```python
from build123d import *

# Parameters (mm, degrees)
SKETCH4_W                      = 69.85
SKETCH4_H                      = 127
BOSS_EXTRUDE4_DEPTH            = 6.35
CBORE_FOR_M3_SHCS1_D           = 3.4
CBORE_FOR_M3_SHCS1_CBORE_D     = 6.5
CBORE_FOR_M3_SHCS1_CBORE_DEPTH = 3.5
SKETCH7_R                      = 1.651
CUT_EXTRUDE1_DEPTH             = 73.748389157
SKETCH16_W                     = 12.7
SKETCH16_H                     = 63.5
BOSS_EXTRUDE6_DEPTH            = 50.8
SKETCH18_W                     = 6.35
SKETCH18_H                     = 63.5
BOSS_EXTRUDE7_DEPTH            = 44.45
CUT_EXTRUDE3_REACH             = 94.294
SKETCH21_R                     = 11.25
CBORE_START                    = 54.15
CBORE_FOR_M3_SHCS3_OUTLINE_R   = 3.25
CBORE_FOR_M3_SHCS3_DEPTH       = 3
CBORE_START_2                  = 50.8
CBORE_FOR_M3_SHCS3_2_OUTLINE_R = 1.7
CBORE_FOR_M3_SHCS3_2_DEPTH     = 3.35
CBORE_FOR_M3_SHCS3_3_OUTLINE_R = 1.7
CBORE_FOR_M3_SHCS3_3_DEPTH     = 6.35
CUT_EXTRUDE5_REACH             = 94.294
CUT_EXTRUDE6_REACH             = 90.502
SKETCH24_W                     = 42.188209008
SKETCH24_H                     = 6.56852392
SKETCH25_W                     = 19.05
SKETCH25_H                     = 40.64
BOSS_EXTRUDE8_DEPTH            = 35.548437
BOSS_EXTRUDE9_DEPTH            = 5
SKETCH32_W                     = 8.128
SKETCH32_H                     = 38.354
CUT_EXTRUDE8_DEPTH             = 1.524
M3_CLEARANCE_HOLE2_D           = 2.8
FILLET6_R                      = 2.54
FILLET9_R                      = 2
FILLET10_R                     = 2
FILLET11_R                     = 2


# Read off the part's stored shape, not the designer's step: CBORE for M3 SHCS3
with BuildPart() as part:
    # Sketch4 → Boss-Extrude4 (new body)
    with BuildSketch(Plane.XY):
        Rectangle(SKETCH4_W, SKETCH4_H)
    extrude(amount=BOSS_EXTRUDE4_DEPTH)

    # CBORE for M3 SHCS1 (through all)
    with Locations(Plane.XY.offset(6.35)):
        with Locations((-10, -24.45), (10, -44.45), (10, -24.45), (-10, -44.45)):
            CounterBoreHole(CBORE_FOR_M3_SHCS1_D / 2, CBORE_FOR_M3_SHCS1_CBORE_D / 2, CBORE_FOR_M3_SHCS1_CBORE_DEPTH)

    # Sketch7 → Cut-Extrude1 (cut, through all)
    with BuildSketch(Plane.XY.offset(6.35)):
        with Locations((-12.5, -34.45)):
            Circle(SKETCH7_R)
        with Locations((12.5, -34.45)):
            Circle(SKETCH7_R)
    extrude(amount=-CUT_EXTRUDE1_DEPTH, mode=Mode.SUBTRACT)

    # Sketch16 → Boss-Extrude6 (add)
    with BuildSketch(Plane.XY.offset(6.35)):
        with Locations((-28.575, 31.75)):
            Rectangle(SKETCH16_W, SKETCH16_H)
        with Locations((28.575, 31.75)):
            Rectangle(SKETCH16_W, SKETCH16_H)
    extrude(amount=BOSS_EXTRUDE6_DEPTH)

    # Sketch18 → Boss-Extrude7 (add)
    with BuildSketch(Plane(origin=(-22.225, 0, 0), x_dir=(0, 0, -1), z_dir=(1, 0, 0))):
        with Locations((-53.975, 31.75)):
            Rectangle(SKETCH18_W, SKETCH18_H)
    extrude(amount=BOSS_EXTRUDE7_DEPTH)

    # Sketch21 → Cut-Extrude3 (cut, up to next)
    with BuildSketch(Plane.XY.offset(57.15), mode=Mode.PRIVATE) as cut_extrude3_sk1:
        with Locations((0, 31.75)):
            Circle(SKETCH21_R)
    cut_extrude3_tool1 = extrude(cut_extrude3_sk1.sketch, amount=-CUT_EXTRUDE3_REACH, mode=Mode.PRIVATE) & part.part
    add(cut_extrude3_tool1.solids().sort_by_distance((0, 31.75, 57.15))[0], mode=Mode.SUBTRACT)

    # CBORE for M3 SHCS3 outline → CBORE for M3 SHCS3 (cut)
    with BuildSketch(Plane.XY.offset(CBORE_START)):
        with Locations((-15.5, 47.25)):
            Circle(CBORE_FOR_M3_SHCS3_OUTLINE_R)
        with Locations((-15.5, 16.25)):
            Circle(CBORE_FOR_M3_SHCS3_OUTLINE_R)
        with Locations((15.5, 47.25)):
            Circle(CBORE_FOR_M3_SHCS3_OUTLINE_R)
        with Locations((15.5, 16.25)):
            Circle(CBORE_FOR_M3_SHCS3_OUTLINE_R)
    extrude(amount=CBORE_FOR_M3_SHCS3_DEPTH, mode=Mode.SUBTRACT)

    # CBORE for M3 SHCS3 2 outline → CBORE for M3 SHCS3 2 (cut)
    with BuildSketch(Plane.XY.offset(CBORE_START_2)):
        with Locations((-15.5, 47.25)):
            Circle(CBORE_FOR_M3_SHCS3_2_OUTLINE_R)
        with Locations((-15.5, 16.25)):
            Circle(CBORE_FOR_M3_SHCS3_2_OUTLINE_R)
        with Locations((15.5, 47.25)):
            Circle(CBORE_FOR_M3_SHCS3_2_OUTLINE_R)
        with Locations((15.5, 16.25)):
            Circle(CBORE_FOR_M3_SHCS3_2_OUTLINE_R)
    extrude(amount=CBORE_FOR_M3_SHCS3_2_DEPTH, mode=Mode.SUBTRACT)

    # CBORE for M3 SHCS3 3 outline → CBORE for M3 SHCS3 3 (cut)
    with BuildSketch(Plane.XY):
        with Locations((0, 31.75)):
            Circle(CBORE_FOR_M3_SHCS3_3_OUTLINE_R)
    extrude(amount=CBORE_FOR_M3_SHCS3_3_DEPTH, mode=Mode.SUBTRACT)

    # Sketch23 → Cut-Extrude5 (cut, up to next)
    with BuildSketch(Plane.XY.offset(57.15), mode=Mode.PRIVATE) as cut_extrude5_sk1:
        with BuildLine():
            Line((-2.53747066, 36.810770012), (-2.53747066, 63.5))
            ThreePointArc((-2.53747066, 63.5), (0, 66.03747066), (2.53747066, 63.5))
            Line((2.53747066, 63.5), (2.53747066, 36.810770012))
            ThreePointArc((2.53747066, 36.810770012), (0, 34.273299352), (-2.53747066, 36.810770012))
        make_face()
    cut_extrude5_tool1 = extrude(cut_extrude5_sk1.sketch, amount=-CUT_EXTRUDE5_REACH, mode=Mode.PRIVATE) & part.part
    add(cut_extrude5_tool1.solids().sort_by_distance((0, 50.155385, 57.15))[0], mode=Mode.SUBTRACT)

    # Sketch24 → Cut-Extrude6 (cut, up to next)
    with BuildSketch(Plane.XY.offset(6.35), mode=Mode.PRIVATE) as cut_extrude6_sk1:
        Rectangle(SKETCH24_W, SKETCH24_H)
    cut_extrude6_tool1 = extrude(cut_extrude6_sk1.sketch, amount=-CUT_EXTRUDE6_REACH, mode=Mode.PRIVATE) & part.part
    add(cut_extrude6_tool1.solids().sort_by_distance((0, 0, 6.35))[0], mode=Mode.SUBTRACT)

    # Sketch25 → Boss-Extrude8 (add)
    with BuildSketch(Plane.ZY.offset(34.925)):
        with Locations((12.777, 31.75)):
            Rectangle(SKETCH25_W, SKETCH25_H)
    extrude(amount=BOSS_EXTRUDE8_DEPTH)

    # Sketch31 → Boss-Extrude9 (add, symmetric)
    with BuildSketch(Plane(origin=(0, 0, 12.777), x_dir=(-1, 0, 0), z_dir=(0, 0, -1))):
        Polygon((34.925, 11.43), (70.4734375, 11.43), (34.925, 0), align=None)
    extrude(amount=BOSS_EXTRUDE9_DEPTH, both=True)

    # Sketch32 → Cut-Extrude8 (cut)
    with BuildSketch(Plane.XY.offset(22.302)):
        with Locations((-55.4734375, 31.75)):
            Rectangle(SKETCH32_W, SKETCH32_H)
    extrude(amount=-CUT_EXTRUDE8_DEPTH, mode=Mode.SUBTRACT)

    # M3 Clearance Hole2 (through all)
    with Locations(Plane.XY.offset(20.778)):
        with Locations((-55.4734375, 31.75)):
            Hole(M3_CLEARANCE_HOLE2_D / 2)

    # Fillet6
    fillet6_edges = [part.edges().sort_by_distance(p)[0] for p in [
        (-34.925, 11.43, 5.5145),
        (-34.925, 11.43, 20.0395),
        (-52.699218512, 11.43, 17.777),
        (-52.699218512, 11.43, 7.777),
    ]]
    fillet(fillet6_edges, radius=FILLET6_R)

    # Fillet9
    # the kernel refuses this fillet: 2 mm, written as the material it takes off along each edge
    with BuildSketch(Plane(origin=(-70.473437, 57.07, 22.302), x_dir=(0, 0, -1), z_dir=(0, -1, 0)), Plane(origin=(-70.473437, 6.43, 3.252), x_dir=(0, 0, 1), z_dir=(0, 1, 0))) as fillet9_piece_1:
        with BuildLine():
            CenterArc((FILLET9_R, FILLET9_R), FILLET9_R, 180, 90)
            Line((0, FILLET9_R), (0, 0))
            Line((0, 0), (FILLET9_R, 0))
        make_face()
    extrude(amount=50.64, mode=Mode.SUBTRACT)
    with BuildSketch(Plane(origin=(-70.473437, 52.07, -1.748), x_dir=(0, -1, 0), z_dir=(0, 0, 1))) as fillet9_piece_2:
        with BuildLine():
            CenterArc((FILLET9_R, FILLET9_R), FILLET9_R, 180, 90)
            Line((0, FILLET9_R), (0, 0))
            Line((0, 0), (FILLET9_R, 0))
        make_face()
    extrude(amount=29.05, mode=Mode.SUBTRACT)

    # Fillet10
    fillet10_edges = [part.edges().sort_by_distance(p)[0] for p in [
        (-34.925, 52.07, 12.777),
    ]]
    fillet(fillet10_edges, radius=FILLET10_R)

    # Fillet11
    fillet11_edges = [part.edges().sort_by_distance(p)[0] for p in [
        (-34.925, 31.48, 3.252),
        (-34.925, 31.48, 22.302),
    ]]
    fillet(fillet11_edges, radius=FILLET11_R)


solid = part.part
```
CAD build for the part. Positions are in the model's coordinates, mm. A direction names the side the tool comes from. Coordinates: 2 decimals unless noted, no trailing zeros. Order: outer loops, then holes, each group sorted by start corner. A loop starts at its lowest first (then second) coordinate and runs counter-clockwise, first axis right, second up. Notation, with made-up numbers: (85, -3.75) - (103, -3.75) arc R25 cw to (103, 22.25) - close; hole circle Ø6 at (75.25, 80). An arc over 180 degrees is marked (long way). Answer in a Markdown table with one row per item.
1. Pull direction Y, two halves, no side cores. Call faces 1 (the face through (-13.247, -44.307, 4.624)), 2 (the face through (-22.225, 31, 28)), 3 (the face through (0, 0, 55)), 4 (the face through (8.43, -45.1, 1.41)): +Y half, -Y half, draft (parallel to the pull), parting line (faces both ways), or undercut.
Answer:
| item | result |
|---|---|
| face 1 | undercut |
| face 2 | draft |
| face 3 | -Y half |
| face 4 | undercut |
2. Flat gauge pins, fed straight in: P1, Ø2, axis at x = 0, z = 51.5, coming from the -Y side; P2, Ø4.5, axis at x = -48.5, y = 4.5, coming from the -Z side; P3, Ø5, axis at y = 51, z = 53.5, coming from the -X side (3 decimals). Where does each tip first touch, or does it go through?
Answer:
| item | result |
|---|---|
| P1 | y = 0 |
| P2 | z = 7.78 |
| P3 | x = -34.925 |
3. Slice it at C-C, the plane z = 35.5. List the corners of the cut face in (x, y) (3 decimals), then the cut area to 3 significant figures.
Answer:
| item | result |
|---|---|
| outline | (-34.925, 0) - (-22.225, 0) - (-22.225, 63.5) - (-34.925, 63.5) - close; (22.225, 0) - (34.925, 0) - (34.925, 63.5) - (22.225, 63.5) - close |
| area | 1,610 mm² |
4. Slice it at B-B, the plane x = 0. List the corners of the cut face in (y, z).
Answer:
| item | result |
|---|---|
| outline | (-63.5, 0) - (-3.28, 0) - (-3.28, 6.35) - (-63.5, 6.35) - close; (0, 50.8) - (20.5, 50.8) - (20.5, 57.15) - (0, 57.15) - close; (3.28, 0) - (30.05, 0) - (30.05, 6.35) - (3.28, 6.35) - close; (33.45, 0) - (63.5, 0) - (63.5, 6.35) - (33.45, 6.35) - close |
5. Drill centre lines: L1, parallel to Y at x = -15.5, z = 56.25; L2, parallel to Y at x = -10, z = 1; L3, parallel to X at y = 16, z = 55 (3 decimals). Where is each one in solid material? Low to high. Write a range as from..to.
Answer:
| item | result |
|---|---|
| L1 | 0..13, 19.5..44, 50.5..63.5 |
| L2 | -63.5..-46.15, -42.75..-26.15, -22.75..-3.28, 3.28..63.5 |
| L3 | -34.925..-18.74, -12.26..12.26, 18.74..34.925 |
6. Slice it at D-D, the plane y = 31.75. Give the number of separate pieces and of enclosed holes in the cut face, then the cut area to 3 significant figures.
Answer:
| item | result |
|---|---|
| separate pieces | 3 |
| enclosed holes | 0 |
| area | 2,470 mm² |
7. Slice it at A-A, the plane y = -24.45. List the corners of the cut face in (x, z) (3 decimals), then the cut area to 3 significant figures.
Answer:
| item | result |
|---|---|
| outline | (-34.925, 0) - (-11.7, 0) - (-11.7, 2.85) - (-13.25, 2.85) - (-13.25, 6.35) - (-34.925, 6.35) - close; (-8.3, 0) - (8.3, 0) - (8.3, 2.85) - (6.75, 2.85) - (6.75, 6.35) - (-6.75, 6.35) - (-6.75, 2.85) - (-8.3, 2.85) - close; (11.7, 0) - (34.925, 0) - (34.925, 6.35) - (13.25, 6.35) - (13.25, 2.85) - (11.7, 2.85) - close |
| area | 379 mm² |
8. 3-axis set-ups, long thin cutter, end or side, ignore diameter. For faces 5 (the face through (-21.094, 0, 3)), 6 (the face through (-43, 6, 7.777)), 7 (the face through (-52, 31, 3.252)), 8 (the face through (2.537, 53, 54)), 9 (the face through (17, 15, 54.15)): which of +Z, -Z, +X, -X, +Y, -Y reach the whole face in a straight line?
Answer:
| item | result |
|---|---|
| face 5 | -Z |
| face 6 | -Z, -X, -Y |
| face 7 | -Z, -X, +Y, -Y |
| face 8 | +Z, +Y |
| face 9 | +Z |
